For this review, use the dimensioned drawing (mm, ordinates from the lowest corner) and the shaded views. Give positions to 0.01 mm unless a question says otherwise; leave off trailing zeros. Order: outer loops, then holes, each group sorted by start corner. A loop starts at its lowest first (then second) coordinate and runs counter-clockwise, first axis right, second up. Notation, with made-up numbers: (-29, 66.25) -> (-10, 66.25) arc R11 cw to (-10, 76.25) -> close; hole circle Ø11 at (-39.5, 38.25). An arc over 180 degrees is marked (long way). Return JSON: item names as keys, results as strings.
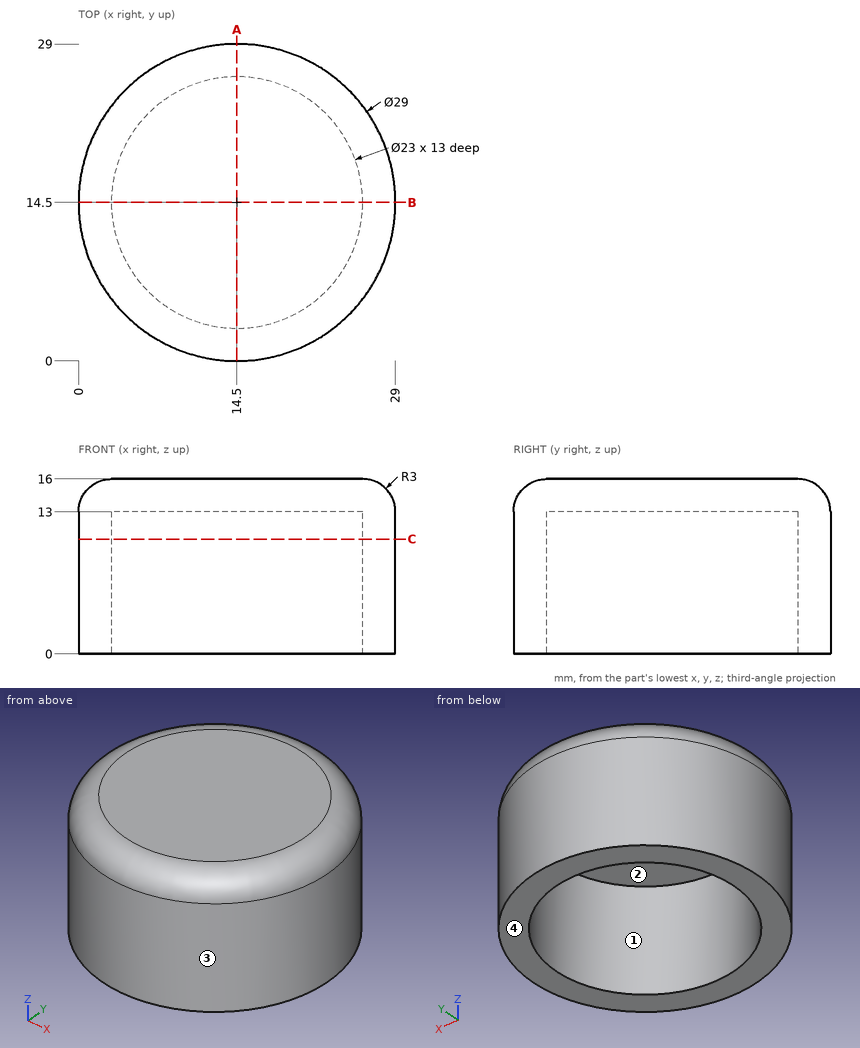
Item 1: Add section C-C (z = 10.5). Give the boundary of the cut face in (x, y).
Result set:
{"outline": "circle Ø29 at (14.5, 14.5); hole circle Ø23 at (14.5, 14.5)"}
Item 2: Mouldability with a two-part tool opening along Y and no side actions: class the marked faces 1, 2, 3 and 4 as released by +Y, released by -Y, zero draft, split by the parting line, or undercut.
Result set:
{"face 1": "undercut", "face 2": "undercut", "face 3": "split by the parting line", "face 4": "zero draft"}
Item 3: Add section A-A (x = 14.5). Give the boundary of the cut face in (y, z), plus the area to 3 significant figures.
Result set:
{"outline": "(0, 0) -> (3, 0) -> (3, 13) -> (26, 13) -> (26, 0) -> (29, 0) -> (29, 13) arc R3 ccw to (26, 16) -> (3, 16) arc R3 ccw to (0, 13) -> close", "area": "161 mm^2"}
Item 4: Wall thickness on L1, parallel to Y at x = 14.5, z = 8.5; L2, parallel to Y at x = 9.75, z = 7; L3, parallel to X at y = 21.5, z = 10.5: over which ranges is each line inside the solid? List them lowest first. Write a range as [from, to].
Result set:
{"L1": "y = [0, 3], [26, 29]", "L2": "y = [0.8, 4.03], [24.97, 28.2]", "L3": "x = [1.8, 5.38], [23.62, 27.2]"}
Item 5: For pin 1 (2 mm diameter, centred on x = 3.5, z = 5.5, fed in from +Y); pin 2 (5 mm diameter, centred on x = 7, z = 2.5, fed in from -Y); pin 3 (1 mm diameter, centred on x = 17, z = 14.5, fed in from -Y), all flat-tipped, find the tip position at first contact; note any pin that passes through.
Result set:
{"pin 1": "stops at y = 25", "pin 2": "stops at y = 0.89", "pin 3": "stops at y = 0.37"}
